Check sheet for the modelled part. Datum: model origin and axes. Units: mm. Give positions to 0.01 mm unless a question says otherwise; leave off trailing zeros. Write each loop counter-clockwise with the first axis right and the second up, starting at its lowest first coordinate (ties: lowest second). Pieces come first, ordered by that corner, then holes. Notation, with made-up numbers: M -39,28 L -27,28 A22 ccw -27,48 Z; hole C 47,52.25 d4. An arc over 180 degrees is marked long. One line per item, written item: value. Start each with the question number.
from build123d import *

# Parameters (mm, degrees)
SKETCH1_W                  = 44.2
SKETCH1_H                  = 123.88
BOSS_EXTRUDE1_DEPTH        = 3.175
F_5_CLEARANCE_HOLE1_D      = 3.4544
F_6_CLEARANCE_HOLE1_D      = 3.7973
FILLET1_R                  = 3.175
F_8_0_199_DIAMETER_HOLE1_D = 5.0546


with BuildPart() as part:
    # Sketch1 → Boss-Extrude1 (new body)
    with BuildSketch(Plane(origin=(0, 0, 0), x_dir=(1, 0, 0), z_dir=(0, 1, 0))):
        with Locations((-12.725, -38.594662694)):
            Rectangle(SKETCH1_W, SKETCH1_H)
    extrude(amount=BOSS_EXTRUDE1_DEPTH)

    # #5 Clearance Hole1 (through all)
    with Locations(Plane(origin=(0, 0, 0), x_dir=(-1, 0, 0), z_dir=(0, -1, 0))):
        with Locations((28.975, 19.845337306), (-3.525, 19.845337306), (-5.3852, -19.737862694), (30.8352, -19.737862694)):
            Hole(F_5_CLEARANCE_HOLE1_D / 2)

    # #6 Clearance Hole1 (through all)
    with Locations(Plane(origin=(0, 3.175, 0), x_dir=(1, 0, 0), z_dir=(0, 1, 0))):
        with Locations((3.025, -97.359662694), (-28.475, -97.359662694)):
            Hole(F_6_CLEARANCE_HOLE1_D / 2)

    # Fillet1
    fillet1_edges = [part.edges().sort_by_distance(p)[0] for p in [
        (-34.825, 1.5875, -23.345337306),
        (9.375, 1.5875, -23.345337306),
        (9.375, 1.5875, 100.534662694),
        (-34.825, 1.5875, 100.534662694),
    ]]
    fillet(fillet1_edges, radius=FILLET1_R)

    # #8 (0.199) Diameter Hole1 (through all)
    with Locations(Plane(origin=(0, 0, 0), x_dir=(-1, 0, 0), z_dir=(0, -1, 0))):
        with Locations((-3.15, -30.684662694), (28.6, -30.684662694), (12.725, -68.784662694)):
            Hole(F_8_0_199_DIAMETER_HOLE1_D / 2)


solid = part.part
1) Material ranges on L1, parallel to X at y = 0.6, z = 18.5 (3 decimals); L2, parallel to Z at x = -28, y = 2.75; L3, parallel to Z at x = 1.5, y = 0.75, recorded low to high. Write a range as from..to.
2) Draft check along X on faces 1 (the cylindrical face through (-33.92, 1.61, -22.39)), 2 (the cylindrical face through (-30.7, 1.6, -19.9)), 3 (the flat face through (-13, 3.175, 38)). Enter one of: released by +X, released by -X, zero draft, split by the parting line, or undercut.
3) Cross-section at A-A (y = 0.85). State how many separate pieces and enclosed holes the cut face has, plus the area to 3 significant figures.
4) Cross-section at B-B (z = 29.5). Record the boundary of the cut face in (x, y) (3 decimals), plus the area to 3 significant figures.
Data:
1. L1: x = -34.825..-32.04, -29.631..4.181, 6.59..9.375
1. L2: z = -23.35..-21.27, -18.42..28.23, 33.14..95.52, 99.2..100.53
1. L3: z = -23.35..28.77, 32.6..96.23, 98.49..100.53
2. face 1: released by -X
2. face 2: undercut
2. face 3: zero draft
3. separate pieces: 1
3. enclosed holes: 9
3. area: 5,350 mm2
4. outline: M -34.825,0 L -30.832,0 L -30.832,3.175 L -34.825,3.175 Z; M -26.368,0 L 0.918,0 L 0.918,3.175 L -26.368,3.175 Z; M 5.382,0 L 9.375,0 L 9.375,3.175 L 5.382,3.175 Z
4. area: 112 mm2
